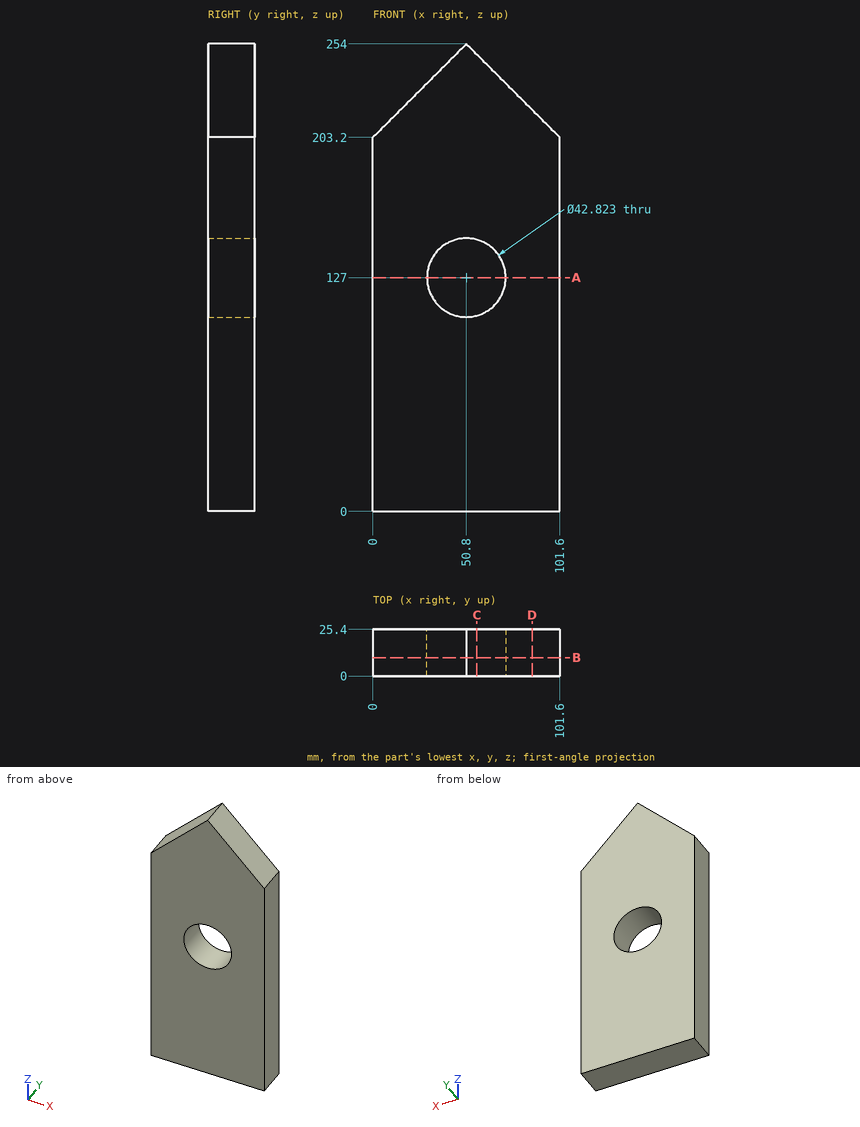
Geometry: see drawing. Coordinates: mm, zero at the bounding-box minimum. Coordinates: 2 decimals unless noted, no trailing zeros. Write each loop counter-clockwise with the first axis right and the second up, starting at its lowest first coordinate (ties: lowest second). Pieces come first, ordered by that corner, then holes.
1) Section D-D on x = 86.5. Output: boundary loops of the cut face in (y, z), and give its area (3 significant figures).
2) Section A-A on z = 127. Output: boundary loops of the cut face in (x, y).
3) Pin query (flat end, axial travel): pin 1 Ø6 at (y, z) = (17, 209) entering from -X; pin 2 Ø6 at (x, y) = (52.5, 10) entering from -Z; pin 3 Ø8 at (x, y) = (80, 20.5) entering from +Z; pin 4 Ø2 at (x, y) = (10, 16) entering from +Z. Return the tip coordinate at first contact, or that it passes through.
4) Section B-B on y = 10. Output: boundary loops of the cut face in (x, z), and give its area (3 significant figures).
5) Section C-C on x = 56.5. Output: boundary loops of the cut face in (y, z).
6) Material intervals for line 1 along Z through (x, y) = (50.8, 16.5); line 2 along Z through (x, y) = (62, 19); line 3 along X through (y, z) = (13.75, 112.5) (1 decimal), sorted ascending.
Check result:
1. outline: (0, 0) - (25.4, 0) - (25.4, 218.3) - (0, 218.3) - close
1. area: 5,540 mm2
2. outline: (0, 0) - (29.39, 0) - (29.39, 25.4) - (0, 25.4) - close; (72.21, 0) - (101.6, 0) - (101.6, 25.4) - (72.21, 25.4) - close
3. pin 1: stops at x = 2.8
3. pin 2: stops at z = 0
3. pin 3: stops at z = 228.8
3. pin 4: stops at z = 214.2
4. outline: (0, 0) - (101.6, 0) - (101.6, 203.2) - (50.8, 254) - (0, 203.2) - close; hole circle Ø42.82 at (50.8, 127)
4. area: 21,800 mm2
5. outline: (0, 0) - (25.4, 0) - (25.4, 106.36) - (0, 106.36) - close; (0, 147.64) - (25.4, 147.64) - (25.4, 248.3) - (0, 248.3) - close
6. line 1: z = 0 to 105.59, 148.41 to 254
6. line 2: z = 0 to 108.75, 145.25 to 242.8
6. line 3: x = 0 to 35, 66.6 to 101.6
